The drawing under review shows one solid part. Ordinate dimensions are in mm from its lowest x, y, z. Coordinates: 2 decimals unless noted, no trailing zeros. Loops run counter-clockwise (first coordinate to the right, second up) from the corner with the lowest first, then second, coordinate; pieces in that order, holes last. Notation, with made-up numbers: (61, 32.5) - (91, 32.5) arc R20 ccw to (91, 40.5) - close; hole circle Ø3 at (75, 12.25). An arc over 180 degrees is marked (long way). Answer as a JSON object with one key per item and string values. Group by question number.
Item 1: We need section D-D (z = 4). Give the boundary of the cut face in (x, y), then the cut area to 3 significant figures.
Item 2: We need section B-B (x = 25). Give the boundary of the cut face in (y, z), then the cut area to 3 significant figures.
Item 3: We need section A-A (z = 25). Give the boundary of the cut face in (x, y), then the cut area to 3 significant figures.
Item 4: To check wall thickness, follow line 1 (Z direction, x = 25, y = 1.55); line 2 (Z direction, x = 27.5, y = 1.7). State the ranges of each line that lie inside material, in increasing order.
Item 5: Clearance check with a flat-ended pin moving along its axis: pin 1 (10.5 mm diameter, centred on x = 25, z = 25, fed in from +Y). State where the tip first meets the part, or that it passes through.
Item 6: We need section C-C (y = 0.75). Give the boundary of the cut face in (x, z), then the cut area to 3 significant figures.
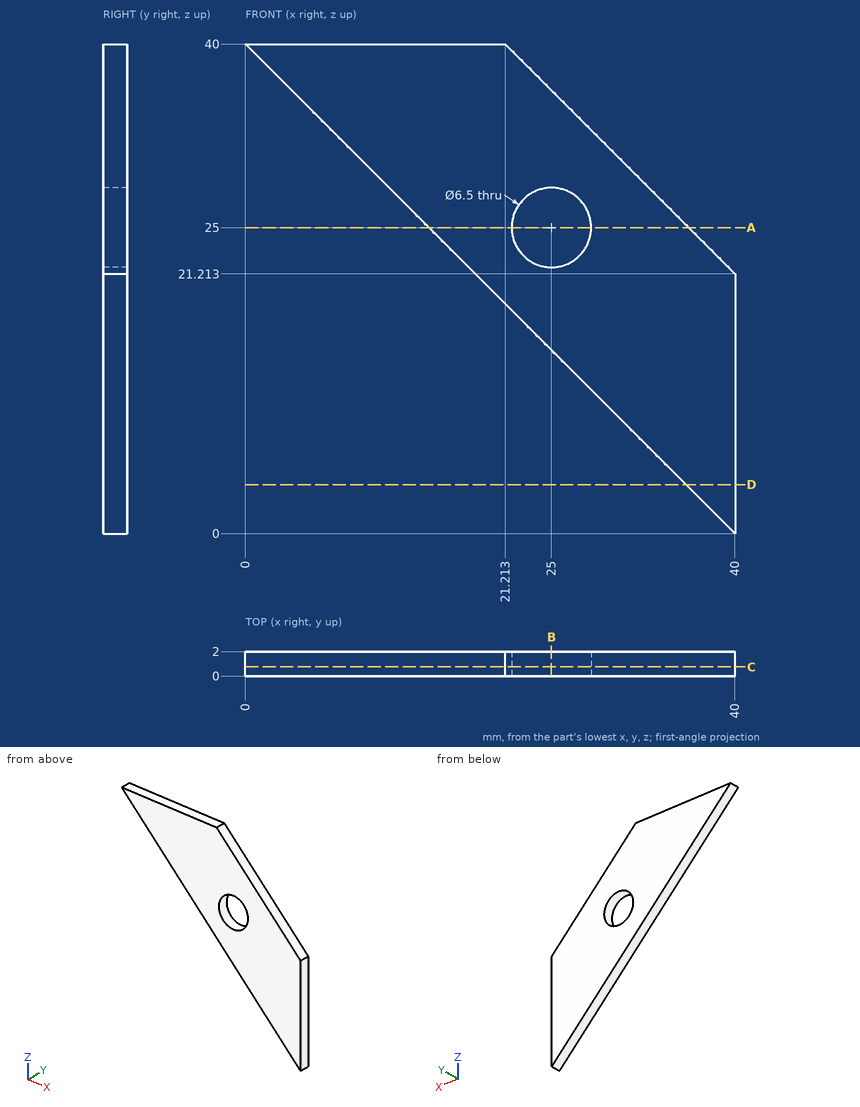
Check sheet entries:
{
 "1": {"outline": "(36, 0) - (40, 0) - (40, 2) - (36, 2) - close", "area": "8.00 mm2"},
 "2": {"outline": "(0, 15) - (2, 15) - (2, 21.75) - (0, 21.75) - close; (0, 28.25) - (2, 28.25) - (2, 36.21) - (0, 36.21) - close", "area": "29.4 mm2"},
 "3": {"outline": "(15, 0) - (21.75, 0) - (21.75, 2) - (15, 2) - close; (28.25, 0) - (36.21, 0) - (36.21, 2) - (28.25, 2) - close", "area": "29.4 mm2"},
 "4": {"line 1": "z = 15 to 21.75, 28.25 to 36.21", "line 2": "z = 12.5 to 22.92, 27.08 to 33.71"},
 "5": {"pin 1": "stops at y = 2"},
 "6": {"outline": "(0, 40) - (40, 0) - (40, 21.21) - (21.21, 40) - close; hole circle Ø6.5 at (25, 25)", "area": "590 mm2"}
}
